Here's the drawing with two shaded views (mm, measured from the low corner). I have some questions. A direction names the side the tool comes from. Coordinates: 2 decimals unless noted, no trailing zeros. Answer as a JSON object with one key per item and string values. Group by question number.
(1) I want a section at C-C, the plane z = 3. State how many separate pieces and enclosed holes the cut face has.
(2) For pin 1 (12.5 mm diameter, centred on x = 25, y = 13.5, fed in from -Z) (1 decimal); pin 2 (3 mm diameter, centred on x = 22.5, y = 14.5, fed in from +Z), each with a flat end and sliding along its axis, tell me the tip position at first contact or that it passes through.
(3) Which directions (+Z, -Z, +X, -X, +Y, -Y) give clear straight access to the entire face, cutting with the end or side of a thin tool? Please do the marked faces 1 and 2.
(4) I need wall thicknesses on line 1 (X direction, y = 6.35, z = 7.75) (1 decimal); line 2 (X direction, y = 8.5, z = 20) (1 decimal); line 3 (X direction, y = 6, z = 19.5) (1 decimal). Which ranges of each line are inside material? Lowest first, please.
(5) If we mould it in two halves opening along X, with no side actions, what happens to the marked faces 3, 4 and 5? For each: pulls with the +X half, pulls with the -X half, needs draft (parallel to the pull), parting line crosses it, or undercut.
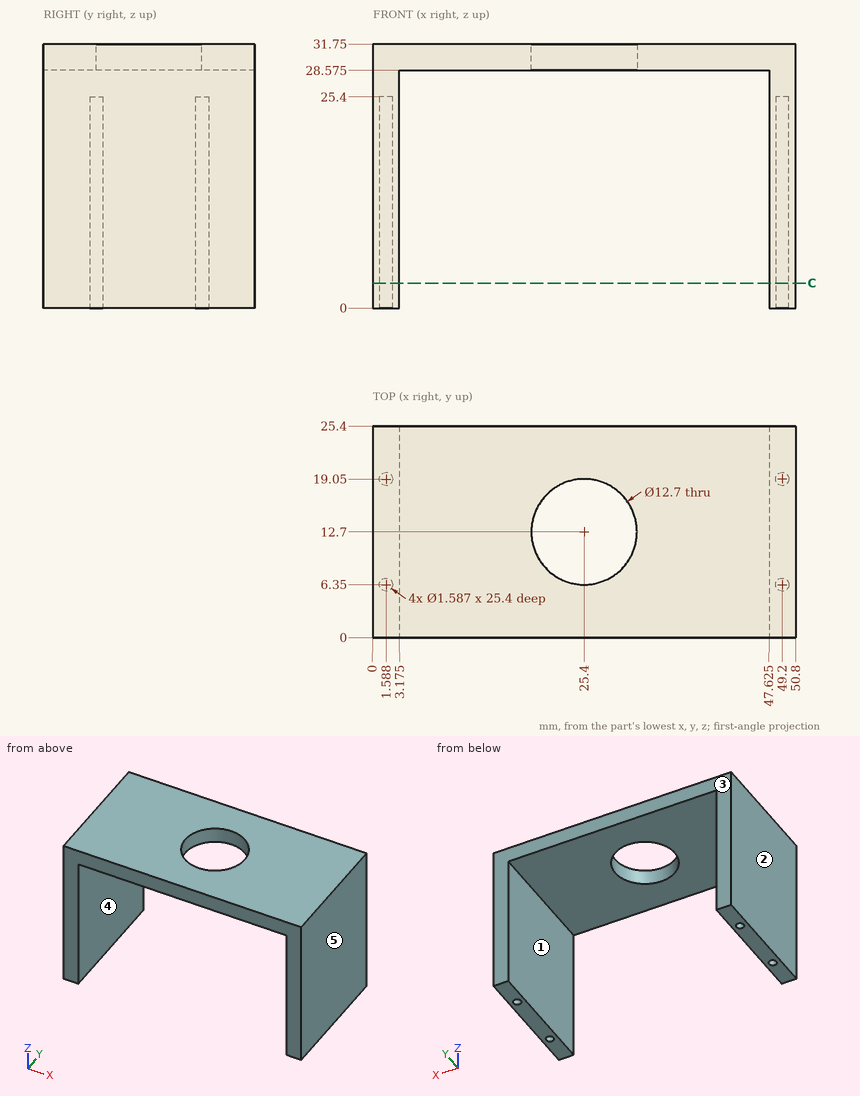
Computed values:
{
 "1": {"separate pieces": "2", "enclosed holes": "4"},
 "2": {"pin 1": "stops at z = 28.6", "pin 2": "passes through"},
 "3": {"face 1": "-Z, +Y, -Y", "face 2": "+Z, -Z, -X, +Y, -Y"},
 "4": {"line 1": "x = 0 to 0.8, 2.4 to 3.2, 47.6 to 48.4, 50 to 50.8", "line 2": "x = 0 to 3.2, 47.6 to 50.8", "line 3": "x = 0 to 0.9, 2.3 to 3.2, 47.6 to 48.5, 49.9 to 50.8"},
 "5": {"face 3": "needs draft", "face 4": "undercut", "face 5": "pulls with the +X half"}
}
